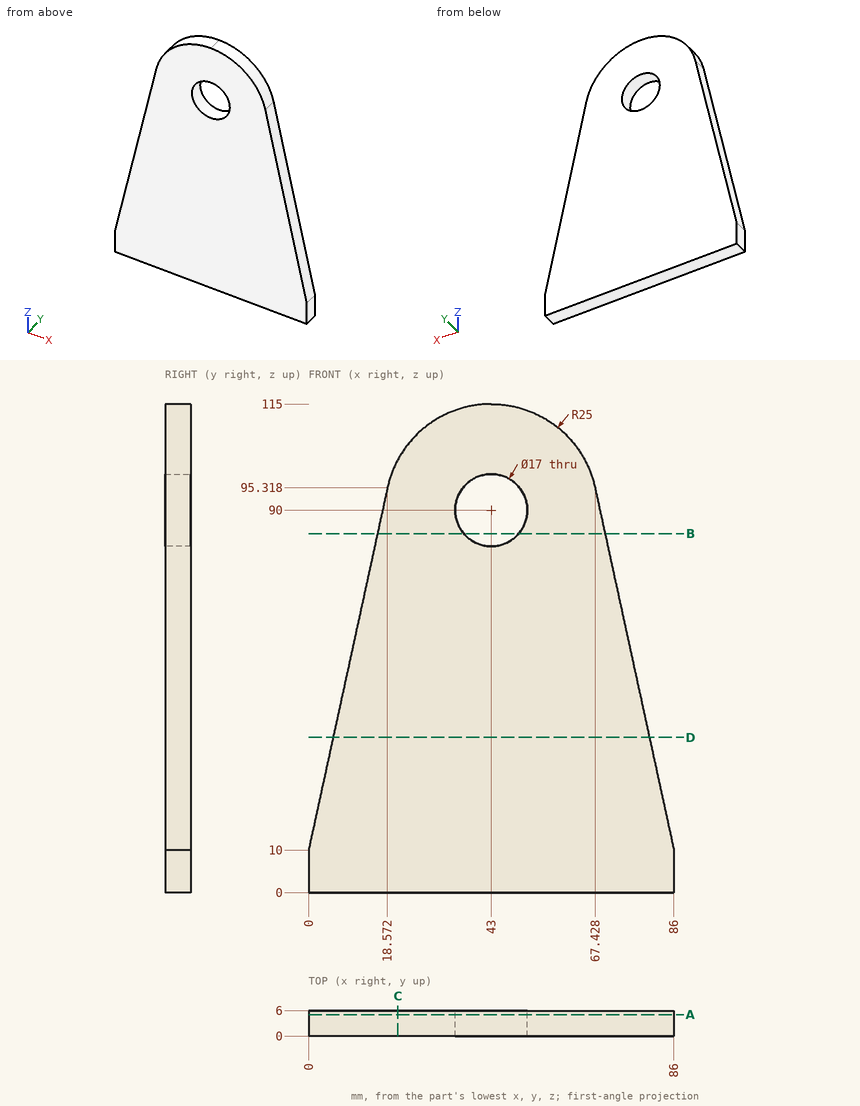
Check sheet for the drawn part. Datum: minimum x, y, z corner. Units: mm. Round coordinates to 2 decimals unless told otherwise and drop trailing zeros. Order: outer loops, then holes, each group sorted by start corner. A loop starts at its lowest first (then second) coordinate and runs counter-clockwise, first axis right, second up.
(1) Cross-section at C-C, the plane x = 21. Enter the section's corners in (y, z) (1 decimal).
(2) Cross-section at B-B, the plane z = 84.5. Enter the section's corners in (x, y), and give its area (3 significant figures).
(3) Cross-section at D-D, the plane z = 36.5. Enter the section's corners in (x, y), and give its area (3 significant figures).
(4) Cross-section at A-A, the plane y = 5.05. Enter the section's corners in (x, z), and give its area (3 significant figures).
(5) Scan lines: probe 1 along Z at (x, y) = (43, 1.2); probe 2 along Z at (x, y) = (37.5, 0.9) (1 decimal); probe 3 along X at (y, z) = (1.55, 90) (1 decimal). Record each from-to range of solid material in increasing order.
(6) Go/stop test with flat-tipped pins: P1, Ø3, axis at y = 5.5, z = 76.5, coming from the +X side; P2, Ø1, axis at x = 47.5, y = 5, coming from the +Z side; P3, Ø12, axis at x = 26.5, z = 102, coming from the -Y side; P4, Ø1, axis at y = 2.5, z = 21.5, coming from the -X side (1 decimal). Record where each tip stops, or that it passes through.
Check sheet entries:
1. outline: (0, 0) - (6, 0) - (6, 101.9) - (0, 101.9) - close
2. outline: (16.22, 0) - (36.52, 0) - (36.52, 6) - (16.22, 6) - close; (49.48, 0) - (69.78, 0) - (69.78, 6) - (49.48, 6) - close
2. area: 244 mm2
3. outline: (5.77, 0) - (80.23, 0) - (80.23, 6) - (5.77, 6) - close
3. area: 447 mm2
4. outline: (0, 0) - (86, 0) - (86, 10) - (67.43, 95.32) arc R25 ccw to (18.57, 95.32) - (0, 10) - close; hole circle Ø17 at (43, 90)
4. area: 7,100 mm2
5. probe 1: z = 0 to 81.5, 98.5 to 115
5. probe 2: z = 0 to 83.5, 96.5 to 114.4
5. probe 3: x = 17.4 to 34.5, 51.5 to 68.6
6. P1: stops at x = 71.85
6. P2: stops at z = 114.68
6. P3: stops at y = 0
6. P4: stops at x = 2.4
